Read the model definition and answer for the solid it produces. Units are mm, in the model's axes. Face numbers are marked on the shaded views. A direction names the side the tool comes from. Coordinates: 2 decimals unless noted, no trailing zeros. Loops run counter-clockwise (first coordinate to the right, second up) from the corner with the lowest first, then second, coordinate; pieces in that order, holes last. Notation, with made-up numbers: M -32,56 L -6,56 A13 ccw -6,67 Z; hole C 5.5,15 d1. An arc over 180 degrees is marked long. One line per item, written item: value. Start each with the question number.
1. The part is cut by section A-A (y = -11.75). Write down the section's boundary in (x, z).
2. The part is cut by section D-D (z = 4.5). Write down the section's boundary in (x, y).
3. The part is cut by section B-B (z = 6.5). Write down the section's boundary in (x, y), then the cut area to 3 significant figures.
4. The part is cut by section C-C (x = -1). Write down the section's boundary in (y, z).
5. For the marked faces 1, 2 and 3, determine the directions among +Z, -Z, +X, -X, +Y, -Y from which every point of the face is accessible in a straight line to the end or side of a thin tool.
6. Flat-ended cylindrical pins translate along their axes: pin 1 (0.6 mm diameter, centred on x = -4.5, y = -9, fed in from +Z); pin 2 (1.2 mm diameter, centred on y = 1.5, z = 8, fed in from -X); pin 3 (2 mm diameter, centred on x = -4, y = 5, fed in from +Z). Find the tip coordinate at first contact, or state that the pin passes through.
7. Consider probe 1 along Y at (x, z) = (6, 8.5); probe 2 along X at (y, z) = (7, 5.75); probe 3 along Y at (x, z) = (-3, 4.75). Determine where each line is inside the solid, lowest interval first.
8. Determine the mould class of the marked faces 4, 5, 6 and 7 for opening direction X: +X half, -X half, draft (parallel to the pull), parting line (faces both ways), or undercut.
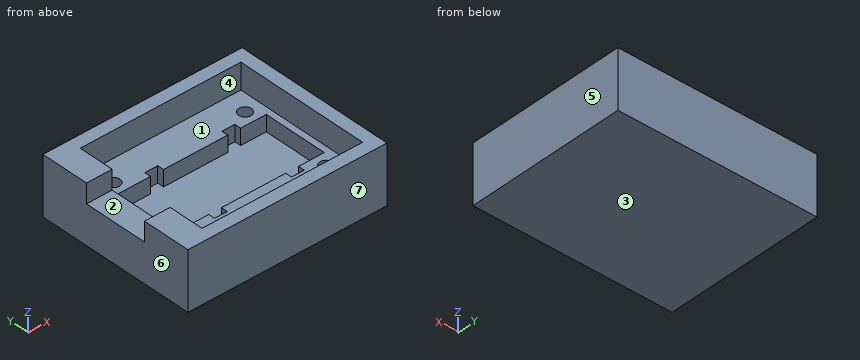
```python
from build123d import *

# Parameters (mm, degrees)
F0_W     = 31
F0_H     = 25
F1_DEPTH = 9
F2_W     = 25
F2_H     = 21
F3_DEPTH = 4
F4_W     = 2
F4_H     = 1
F4_W_2   = 1
F4_H_2   = 10
F5_DEPTH = 6.5
F6_R     = 1
F7_DEPTH = 2
F8_DEPTH = 1
F9_DEPTH = 2


with BuildPart() as f1:
    # F0 (on Top) → F1 (new body)
    with BuildSketch(Plane.XY):
        with Locations((5.1452719867, -1.972973533)):
            Rectangle(F0_W, F0_H)
    extrude(amount=F1_DEPTH)

    # F2 (on face) → F3 (cut)
    with BuildSketch(Plane.XY.offset(9)):
        with Locations((6.1452719867, -1.972973533)):
            Rectangle(F2_W, F2_H)
    extrude(amount=-F3_DEPTH, mode=Mode.SUBTRACT)

    # F4 (on face) → F5 (cut)
    with BuildSketch(Plane.XY.offset(9)):
        with Locations((0.6452719867, 3.527026467)):
            Rectangle(F4_W, F4_H)
        with Locations((12.6452719867, 3.527026467)):
            Rectangle(F4_W, F4_H)
        with Locations((0.6452719867, -7.472973533)):
            Rectangle(F4_W, F4_H)
        with Locations((12.6452719867, -7.472973533)):
            Rectangle(F4_W, F4_H)
        with Locations((17.1452719867, -1.972973533)):
            Rectangle(F4_W_2, F4_H_2)
        Polygon((1.6452719867, 3.027026467), (-0.3547280133, 3.027026467), (-6.3547280133, 3.027026467), (-6.3547280133, -6.972973533), (-0.3547280133, -6.972973533), (1.6452719867, -6.972973533), (11.6452719867, -6.972973533), (13.6452719867, -6.972973533), (16.6452719867, -6.972973533), (16.6452719867, 3.027026467), (13.6452719867, 3.027026467), (11.6452719867, 3.027026467), align=None)
    extrude(amount=-F5_DEPTH, mode=Mode.SUBTRACT)

    # F6 (on face) → F7 (cut)
    with BuildSketch(Plane.XY.offset(5)):
        with Locations((-4.3547280133, 5.027026467)):
            Circle(F6_R)
        with Locations((16.1452719867, 5.027026467)):
            Circle(F6_R)
        with Locations((-4.3547280133, -8.972973533)):
            Circle(F6_R)
        with Locations((16.1452719867, -8.972973533)):
            Circle(F6_R)
    extrude(amount=-F7_DEPTH, mode=Mode.SUBTRACT)

    # F4 (on face) → F8 (cut)
    with BuildSketch(Plane.XY.offset(9)):
        Polygon((-0.3547280133, 3.027026467), (-10.3547280133, 3.027026467), (-10.3547280133, -6.972973533), (-0.3547280133, -6.972973533), (1.6452719867, -6.972973533), (11.6452719867, -6.972973533), (13.6452719867, -6.972973533), (16.6452719867, -6.972973533), (16.6452719867, 3.027026467), (13.6452719867, 3.027026467), (11.6452719867, 3.027026467), (1.6452719867, 3.027026467), align=None)
        with Locations((0.6452719867, 3.527026467)):
            Rectangle(F4_W, F4_H)
        with Locations((0.6452719867, -7.472973533)):
            Rectangle(F4_W, F4_H)
        with Locations((12.6452719867, 3.527026467)):
            Rectangle(F4_W, F4_H)
        with Locations((12.6452719867, -7.472973533)):
            Rectangle(F4_W, F4_H)
        with Locations((17.1452719867, -1.972973533)):
            Rectangle(F4_W_2, F4_H_2)
    extrude(amount=-F8_DEPTH, mode=Mode.SUBTRACT)

    # F9 (cut): a face of the model
    f9_faces = [f1.faces().sort_by_distance(p)[0] for p in [
        (-8.3547280133, -1.972973533, 8),
    ]]
    extrude(f9_faces, amount=-F9_DEPTH, mode=Mode.SUBTRACT)


solid = f1.part
```
Answer block:
1. outline: M -10.35,0 L 20.65,0 L 20.65,9 L 18.65,9 L 18.65,5 L -6.35,5 L -6.35,9 L -10.35,9 Z
2. outline: M -10.35,-14.47 L 20.65,-14.47 L 20.65,10.53 L -10.35,10.53 Z; hole M -6.35,-6.97 L -0.35,-6.97 L -0.35,-7.97 L 1.65,-7.97 L 1.65,-6.97 L 11.65,-6.97 L 11.65,-7.97 L 13.65,-7.97 L 13.65,-6.97 L 17.65,-6.97 L 17.65,3.03 L 13.65,3.03 L 13.65,4.03 L 11.65,4.03 L 11.65,3.03 L 1.65,3.03 L 1.65,4.03 L -0.35,4.03 L -0.35,3.03 L -6.35,3.03 Z; hole C -4.35,-8.97 d2; hole C -4.35,5.03 d2; hole C 16.15,-8.97 d2; hole C 16.15,5.03 d2
3. outline: M -10.35,-14.47 L 20.65,-14.47 L 20.65,10.53 L -10.35,10.53 L -10.35,3.03 L -6.35,3.03 L -6.35,8.53 L 18.65,8.53 L 18.65,-12.47 L -6.35,-12.47 L -6.35,-6.97 L -10.35,-6.97 Z
3. area: 210 mm2
4. outline: M -14.47,0 L 10.53,0 L 10.53,9 L 8.53,9 L 8.53,5 L 3.03,5 L 3.03,2.5 L -6.97,2.5 L -6.97,5 L -12.47,5 L -12.47,9 L -14.47,9 Z
5. face 1: +Z
5. face 2: +Z, -X
5. face 3: -Z, +X, -X, +Y, -Y
6. pin 1: stops at z = 3
6. pin 2: stops at x = 18.65
6. pin 3: stops at z = 5
7. probe 1: y = -14.47 to -12.47, 8.53 to 10.53
7. probe 2: x = -10.35 to -6.35, 18.65 to 20.65
7. probe 3: y = -14.47 to -6.97, 3.03 to 10.53
8. face 4: undercut
8. face 5: +X half
8. face 6: -X half
8. face 7: draft
